Autodesk Inventor part; units mm, degrees
ref_plane "YZ Plane" through (0, 0, 0) normal (1, 0, 0) x (0, 1, 0)
ref_plane "XZ Plane" through (0, 0, 0) normal (0, 1, 0) x (-1, 0, 0)
ref_plane "XY Plane" through (0, 0, 0) normal (0, 0, 1) x (1, 0, 0)
sketch "Sketch1" plane through (0, 0, 0) normal (0, 0, 1) x (1, 0, 0)
  line L0 (97.5839, -20.2585) -> (97.5839, -84.5585) construction
  line L1 (97.5839, -52.4085) -> (19.6066, -52.4085)
  line L2 (622.5839, -227.4085) -> (-427.4161, -227.4085)
  line L3 (-427.4161, -227.4085) -> (-427.4161, 122.5915)
  line L4 (-427.4161, 122.5915) -> (622.5839, 122.5915)
  line L5 (622.5839, 122.5915) -> (622.5839, -227.4085)
  line L6 (622.5839, -227.4085) -> (-427.4161, 122.5915) construction
  line L7 (-427.4161, -227.4085) -> (622.5839, 122.5915) construction
  line L8 (-402.4161, 97.5915) -> (597.5839, 97.5915)
  line L9 (597.5839, 97.5915) -> (597.5839, -202.4085)
  line L10 (597.5839, -202.4085) -> (-402.4161, -202.4085)
  line L11 (-402.4161, -202.4085) -> (-402.4161, 97.5915)
  line L12 (-402.4161, 97.5915) -> (597.5839, -202.4085) construction
  line L13 (597.5839, 97.5915) -> (-402.4161, -202.4085) construction
  circle A0 centre (-417.4161, -217.4085) radius 3
  circle A1 centre (-159.9161, -217.4085) radius 3
  circle A2 centre (97.5839, 112.5915) radius 3
  circle A3 centre (-159.9161, 112.5915) radius 3
  circle A4 centre (-417.4161, 112.5915) radius 3
  circle A5 centre (355.0839, 112.5915) radius 3
  circle A6 centre (612.5839, 112.5915) radius 3
  circle A7 centre (612.5839, -217.4085) radius 3
  circle A8 centre (355.0839, -217.4085) radius 3
  circle A9 centre (97.5839, -217.4085) radius 3
  point P0 (0, 0)
  dimension "d0" = 1050
  dimension "d1" = 350
  dimension "d6" = 1000
  dimension "d7" = 300
extrude "Extrusion2" add sketch "Sketch1" along normal blind 4
properties part number "PrimaryCoilAluminiumLayer" material "Silver"
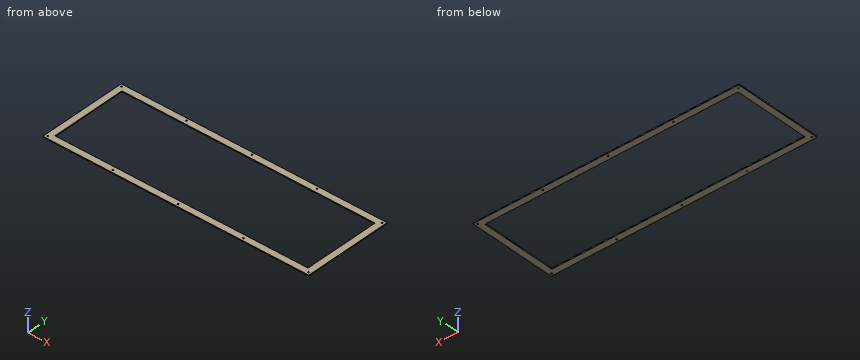
Here's how the part is built. I have some questions about the finished solid (model axes, mm). Give positions to 0.01 mm unless a question says otherwise; leave off trailing zeros. Order: outer loops, then holes, each group sorted by start corner. A loop starts at its lowest first (then second) coordinate and runs counter-clockwise, first axis right, second up. Notation, with made-up numbers: (-21.75, 19.5) -> (23.25, 19.5) arc R35 ccw to (23.25, 51.5) -> close; hole circle Ø2 at (22, -28). An arc over 180 degrees is marked (long way). Use CSV: the item, a comma, the result in double quotes. Start each with the question number.
Item 1: Suppose I cut it at C-C (z = 0.8). Give the number of separate pieces and of enclosed holes in the cut face, and give its area (3 significant figures).
Item 2: If I drill on probe 1 along X at (y, z) = (-24, 3.45); probe 2 along Y at (x, z) = (194.5, 3.2), over which ranges is the centre line in solid material (lowest first)? Write a range as [from, to].
Item 3: Suppose I cut it at B-B (x = -246.5). List the corners of the cut face in (y, z) for me.
Item 4: Suppose I cut it at A-A (y = 26.5). List the corners of the cut face in (x, z) for me, and give its area (3 significant figures).
Answer block:
1,separate pieces,"1"
1,enclosed holes,"11"
1,area,"67,200 mm^2"
2,probe 1,"x = [-427.42, -402.42], [597.58, 622.58]"
2,probe 2,"y = [-227.41, -202.41], [97.59, 122.59]"
3,outline,"(-227.41, 0) -> (-202.41, 0) -> (-202.41, 4) -> (-227.41, 4) -> close; (97.59, 0) -> (122.59, 0) -> (122.59, 4) -> (97.59, 4) -> close"
4,outline,"(-427.42, 0) -> (-402.42, 0) -> (-402.42, 4) -> (-427.42, 4) -> close; (597.58, 0) -> (622.58, 0) -> (622.58, 4) -> (597.58, 4) -> close"
4,area,"200 mm^2"
